The model under review builds one solid part; all positions refer to its coordinate system, in mm. Face numbers are marked on the shaded views. A direction names the side the tool comes from. Coordinates: 2 decimals unless noted, no trailing zeros. Write each loop counter-clockwise with the first axis right and the second up, starting at its lowest first coordinate (ties: lowest second). Pieces come first, ordered by that corner, then holes.
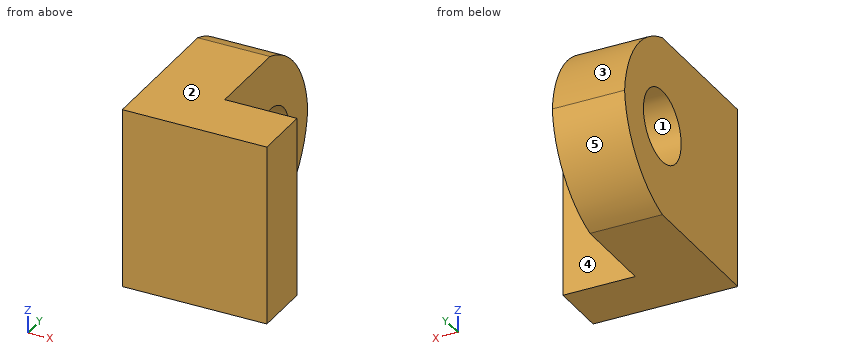
```python
from build123d import *

# Parameters (mm, degrees)
CROQUIS1_W              = 20
CROQUIS1_H              = 25
SALIENTE_EXTRUIR1_DEPTH = 30
CROQUIS2_W              = 10
CROQUIS2_H              = 22
CORTAR_EXTRUIR1_DEPTH   = 30
CORTAR_EXTRUIR3_DEPTH   = 30
CROQUIS7_R              = 5
CORTAR_EXTRUIR4_DEPTH   = 30


with BuildPart() as part:
    # Croquis1 → Saliente-Extruir1 (new body)
    with BuildSketch(Plane(origin=(0, 0, 0), x_dir=(1, 0, 0), z_dir=(0, 1, 0))):
        with Locations((10, -12.5)):
            Rectangle(CROQUIS1_W, CROQUIS1_H)
    extrude(amount=SALIENTE_EXTRUIR1_DEPTH)

    # Croquis2 → Cortar-Extruir1 (cut)
    with BuildSketch(Plane.XY.offset(25)):
        with Locations((15, 19)):
            Rectangle(CROQUIS2_W, CROQUIS2_H)
    extrude(amount=-CORTAR_EXTRUIR1_DEPTH, mode=Mode.SUBTRACT)

    # Croquis6 → Cortar-Extruir3 (cut)
    with BuildSketch(Plane(origin=(10, 0, 0), x_dir=(0, 0, -1), z_dir=(1, 0, 0))):
        with BuildLine():
            Line((-25, 30), (-25, 20))
            ThreePointArc((-25, 20), (-20.308873363, 26.948591704), (-12.5, 30))
            Line((-12.5, 30), (-25, 30))
        make_face()
        with BuildLine():
            ThreePointArc((-12.5, 30), (-4.691126637, 26.948591704), (0, 20))
            Line((0, 20), (0, 30))
            Line((0, 30), (-12.5, 30))
        make_face()
    extrude(amount=-CORTAR_EXTRUIR3_DEPTH, mode=Mode.SUBTRACT)

    # Croquis7 → Cortar-Extruir4 (cut)
    with BuildSketch(Plane(origin=(10, 0, 0), x_dir=(0, 0, -1), z_dir=(1, 0, 0))):
        with Locations((-12.5, 20)):
            Circle(CROQUIS7_R)
    extrude(amount=-CORTAR_EXTRUIR4_DEPTH, mode=Mode.SUBTRACT)


solid = part.part
```
Item 1: Take a section at A-A, the plane z = 10.25. Write out the cut boundary in (x, y).
Solved:
outline: (0, 0) - (20, 0) - (20, 8) - (10, 8) - (10, 15.53) - (0, 15.53) - close; (0, 24.47) - (10, 24.47) - (10, 29.66) - (0, 29.66) - close
Item 2: Take a section at D-D, the plane z = 16. Write out the cut boundary in (x, y), plus the area to 3 significant figures.
Solved:
outline: (0, 0) - (20, 0) - (20, 8) - (10, 8) - (10, 16.43) - (0, 16.43) - close; (0, 23.57) - (10, 23.57) - (10, 29.3) - (0, 29.3) - close
area: 302 mm2
Item 3: Take a section at B-B, the plane y = 23.5. Write out the cut boundary in (x, z), plus the area to 3 significant figures.
Solved:
outline: (0, 1.6) - (10, 1.6) - (10, 8.93) - (0, 8.93) - close; (0, 16.07) - (10, 16.07) - (10, 23.4) - (0, 23.4) - close
area: 147 mm2
Item 4: Machinability: for the marked faces 4 and 5, which of the approach directions +Z, -Z, +X, -X, +Y, -Y give a long, thin tool a straight path to every point of the face, cutting with its end or side? Answer none if there is none.
Solved:
face 4: +Z, -Z, +X, +Y
face 5: -Z, +X, -X, +Y
Item 5: Take a section at C-C, the plane x = 3.5. Write out the cut boundary in (y, z), plus the area to 3 significant figures.
Solved:
outline: (0, 0) - (20, 0) arc R14.08 ccw to (30, 12.5) arc R14.08 ccw to (20, 25) - (0, 25) - close; hole circle Ø10 at (20, 12.5)
area: 601 mm2
Item 6: Mouldability with a two-part tool opening along Y and no side actions: class the marked faces 1, 2 and 3 as pulls with the +Y half, pulls with the -Y half, needs draft (parallel to the pull), parting line crosses it, or undercut.
Solved:
face 1: undercut
face 2: needs draft
face 3: pulls with the +Y half
Item 7: To check wall thickness, follow line 1 along Y through (x, z) = (6.25, 12.5); line 2 along Y through (x, z) = (11, 13.5); line 3 along X through (y, z) = (14.25, 6.5). State the ranges of each line that lie inside material, in increasing order.
Solved:
line 1: y = 0 to 15, 25 to 30
line 2: y = 0 to 8
line 3: x = 0 to 10
Item 8: For pin 1 (8 mm diameter, centred on x = 17, z = 16, fed in from +Y); pin 2 (11.5 mm diameter, centred on y = 20, z = 12.5, fed in from +X); pin 3 (8 mm diameter, centred on x = 8, z = 18, fed in from +Y), all flat-tipped, find the tip position at first contact; note any pin that passes through.
Solved:
pin 1: stops at y = 8
pin 2: stops at x = 10
pin 3: stops at y = 29.81
